from build123d import *

# Parameters (mm, degrees)
BOSS_EXTRUDE1_DEPTH = 15
FILLET1_R           = 30
FILLET2_R           = 6
SKETCH3_W           = 30.5
SKETCH3_H           = 15.5
CUT_EXTRUDE2_DEPTH  = 820.456527218
SKETCH6_W           = 15
SKETCH6_H           = 30
BOSS_EXTRUDE2_DEPTH = 10
SKETCH7_W           = 15
SKETCH7_H           = 15
CUT_EXTRUDE5_DEPTH  = 820.456527218
FILLET4_R           = 6.5
SKETCH9_W           = 75
SKETCH9_H           = 115
BOSS_EXTRUDE3_DEPTH = 15
SKETCH8_W           = 21
SKETCH8_H           = 11
CUT_EXTRUDE6_DEPTH  = 890.119789455
CUT_EXTRUDE7_DEPTH  = 15
SKETCH11_W          = 25
SKETCH11_H          = 50
CUT_EXTRUDE8_DEPTH  = 15
SKETCH5_R           = 2.5
CUT_EXTRUDE4_DEPTH  = 890.119789455
FILLET5_R           = 20
FILLET6_R           = 10
CHAMFER1_SIZE       = 1
SKETCH12_W          = 16
SKETCH12_H          = 11
CUT_EXTRUDE9_DEPTH  = 890.119789455
SKETCH14_W          = 223.5
SKETCH14_H          = 10
CUT_EXTRUDE11_DEPTH = 15
FILLET8_R           = 5
SKETCH15_R          = 2
CUT_EXTRUDE12_DEPTH = 890.119789455
SKETCH16_R          = 2
CUT_EXTRUDE13_DEPTH = 890.119789455
SKETCH17_R          = 2
CUT_EXTRUDE14_DEPTH = 890.119789455
BOSS_EXTRUDE4_DEPTH = 15
FILLET9_R           = 10
FILLET10_R          = 3
SKETCH19_R          = 4.25
CUT_EXTRUDE15_DEPTH = 932.739770537


with BuildPart() as part:
    # Sketch1 → Boss-Extrude1 (new body)
    with BuildSketch(Plane(origin=(0, 0, 0), x_dir=(0, 0, -1), z_dir=(1, 0, 0))):
        Polygon((-678, 0), (0, 0), (0, 460), (75, 460), (75, -69), (-678, -69), align=None)
    extrude(amount=BOSS_EXTRUDE1_DEPTH)

    # Fillet1
    fillet1_edges = [part.edges().sort_by_distance(p)[0] for p in [
        (7.5, -69, -75),
    ]]
    fillet(fillet1_edges, radius=FILLET1_R)

    # Fillet2
    fillet2_edges = [part.edges().sort_by_distance(p)[0] for p in [
        (7.5, 0, 0),
    ]]
    fillet(fillet2_edges, radius=FILLET2_R)

    # Sketch3 → Cut-Extrude2 (cut, through all)
    with BuildSketch(Plane.ZY):
        with Locations((-15.25, 213.5)):
            Rectangle(SKETCH3_W, SKETCH3_H)
    extrude(amount=-CUT_EXTRUDE2_DEPTH, mode=Mode.SUBTRACT)

    # Sketch6 → Boss-Extrude2 (add)
    with BuildSketch(Plane.XY):
        with Locations((7.5, 445)):
            Rectangle(SKETCH6_W, SKETCH6_H)
        with Locations((7.5, 145)):
            Rectangle(SKETCH6_W, SKETCH6_H)
    extrude(amount=BOSS_EXTRUDE2_DEPTH)

    # Sketch7 → Cut-Extrude5 (cut, through all)
    with BuildSketch(Plane.ZY):
        with Locations((-7.5, 198.25)):
            Rectangle(SKETCH7_W, SKETCH7_H)
    extrude(amount=-CUT_EXTRUDE5_DEPTH, mode=Mode.SUBTRACT)

    # Fillet4
    fillet4_edges = [part.edges().sort_by_distance(p)[0] for p in [
        (7.5, 190.75, -15),
    ]]
    fillet(fillet4_edges, radius=FILLET4_R)

    # Sketch9 → Boss-Extrude3 (add)
    with BuildSketch(Plane(origin=(15, 0, 0), x_dir=(0, 0, -1), z_dir=(1, 0, 0))):
        with Locations((37.5, 517.5)):
            Rectangle(SKETCH9_W, SKETCH9_H)
    extrude(amount=-BOSS_EXTRUDE3_DEPTH)

    # Sketch8 → Cut-Extrude6 (cut, through all)
    with BuildSketch(Plane(origin=(15, 0, 0), x_dir=(0, 0, -1), z_dir=(1, 0, 0))):
        with Locations((60, 455)):
            Rectangle(SKETCH8_W, SKETCH8_H)
    extrude(amount=-CUT_EXTRUDE6_DEPTH, mode=Mode.SUBTRACT)

    # Sketch10 → Cut-Extrude7 (cut)
    with BuildSketch(Plane(origin=(15, 0, 0), x_dir=(0, 0, -1), z_dir=(1, 0, 0))):
        Polygon((45, 575), (75, 475), (75, 575), align=None)
    extrude(amount=-CUT_EXTRUDE7_DEPTH, mode=Mode.SUBTRACT)

    # Sketch11 → Cut-Extrude8 (cut)
    with BuildSketch(Plane(origin=(15, 0, 0), x_dir=(0, 0, -1), z_dir=(1, 0, 0))):
        with Locations((27.5, 520)):
            Rectangle(SKETCH11_W, SKETCH11_H)
    extrude(amount=-CUT_EXTRUDE8_DEPTH, mode=Mode.SUBTRACT)

    # Sketch5 → Cut-Extrude4 (cut, through all)
    with BuildSketch(Plane.ZY):
        with Locations((-60, 431)):
            Circle(SKETCH5_R)
    extrude(amount=-CUT_EXTRUDE4_DEPTH, mode=Mode.SUBTRACT)

    # Fillet5
    fillet5_edges = [part.edges().sort_by_distance(p)[0] for p in [
        (7.5, 575, -45),
        (7.5, 475, -75),
    ]]
    fillet(fillet5_edges, radius=FILLET5_R)

    # Fillet6
    fillet6_edges = [part.edges().sort_by_distance(p)[0] for p in [
        (7.5, 495, -15),
        (7.5, 545, -15),
        (7.5, 545, -40),
        (7.5, 495, -40),
    ]]
    fillet(fillet6_edges, radius=FILLET6_R)

    # Chamfer1
    chamfer1_edges = [part.edges().sort_by_distance(p)[0] for p in [
        (7.5, 430, 10),
        (7.5, 460, 10),
        (7.5, 130, 10),
        (7.5, 160, 10),
    ]]
    chamfer(chamfer1_edges, length=CHAMFER1_SIZE)

    # Sketch12 → Cut-Extrude9 (cut, through all)
    with BuildSketch(Plane(origin=(15, 0, 0), x_dir=(0, 0, -1), z_dir=(1, 0, 0))):
        with Locations((27.5, -58.5)):
            Rectangle(SKETCH12_W, SKETCH12_H)
    extrude(amount=-CUT_EXTRUDE9_DEPTH, mode=Mode.SUBTRACT)

    # Sketch14 → Cut-Extrude11 (cut)
    with BuildSketch(Plane(origin=(15, 0, 0), x_dir=(0, 0, -1), z_dir=(1, 0, 0))):
        with Locations((-491.25, -5)):
            Rectangle(SKETCH14_W, SKETCH14_H)
        with Locations((-192.75, -5)):
            Rectangle(SKETCH14_W, SKETCH14_H)
    extrude(amount=-CUT_EXTRUDE11_DEPTH, mode=Mode.SUBTRACT)

    # Fillet8
    fillet8_edges = [part.edges().sort_by_distance(p)[0] for p in [
        (7.5, -10, 603),
        (7.5, -10, 379.5),
        (7.5, -10, 81),
        (7.5, -10, 304.5),
    ]]
    fillet(fillet8_edges, radius=FILLET8_R)

    # Sketch15 → Cut-Extrude12 (cut, through all)
    with BuildSketch(Plane(origin=(15, 0, 0), x_dir=(0, 0, -1), z_dir=(1, 0, 0))):
        with Locations((-0.707106781, 129.292893219)):
            Circle(SKETCH15_R)
        with Locations((-0.707106781, 160.707106781)):
            Circle(SKETCH15_R)
        with Locations((-0.707106781, 429.292893219)):
            Circle(SKETCH15_R)
        with Locations((-0.707106781, 460.707106781)):
            Circle(SKETCH15_R)
    extrude(amount=-CUT_EXTRUDE12_DEPTH, mode=Mode.SUBTRACT)

    # Sketch16 → Cut-Extrude13 (cut, through all)
    with BuildSketch(Plane(origin=(15, 0, 0), x_dir=(0, 0, -1), z_dir=(1, 0, 0))):
        with Locations((50.207106781, 450.207106781)):
            Circle(SKETCH16_R)
        with Locations((50.207106781, 459.792893219)):
            Circle(SKETCH16_R)
        with Locations((69.792893219, 459.792893219)):
            Circle(SKETCH16_R)
        with Locations((69.792893219, 450.207106781)):
            Circle(SKETCH16_R)
    extrude(amount=-CUT_EXTRUDE13_DEPTH, mode=Mode.SUBTRACT)

    # Sketch17 → Cut-Extrude14 (cut, through all)
    with BuildSketch(Plane(origin=(15, 0, 0), x_dir=(0, 0, -1), z_dir=(1, 0, 0))):
        with Locations((29.792893219, 206.457106781)):
            Circle(SKETCH17_R)
        with Locations((29.792893219, 220.542893219)):
            Circle(SKETCH17_R)
    extrude(amount=-CUT_EXTRUDE14_DEPTH, mode=Mode.SUBTRACT)

    # Sketch18 → Boss-Extrude4 (add)
    with BuildSketch(Plane(origin=(15, 0, 0), x_dir=(0, 0, -1), z_dir=(1, 0, 0))):
        with BuildLine():
            Line((-678, -69), (-733, -69))
            Line((-733, -69), (-733, -7))
            Line((-733, -7), (-725.5, -7))
            Line((-725.5, -7), (-720.55324034, -25.378780397))
            ThreePointArc((-720.55324034, -25.378780397), (-708, -35), (-695.44675966, -25.378780397))
            Line((-695.44675966, -25.378780397), (-690.5, -7))
            Line((-690.5, -7), (-678, -7))
            Line((-678, -7), (-678, -69))
        make_face()
    extrude(amount=-BOSS_EXTRUDE4_DEPTH)

    # Fillet9
    fillet9_edges = [part.edges().sort_by_distance(p)[0] for p in [
        (7.5, -69, 733),
    ]]
    fillet(fillet9_edges, radius=FILLET9_R)

    # Fillet10
    fillet10_edges = [part.edges().sort_by_distance(p)[0] for p in [
        (7.5, -7, 733),
        (7.5, -7, 725.5),
        (7.5, -7, 690.5),
    ]]
    fillet(fillet10_edges, radius=FILLET10_R)

    # Sketch19 → Cut-Extrude15 (cut, through all)
    with BuildSketch(Plane(origin=(15, 0, 0), x_dir=(0, 0, -1), z_dir=(1, 0, 0))):
        with Locations((-513, -34)):
            Circle(SKETCH19_R)
        with Locations((-363, -34)):
            Circle(SKETCH19_R)
    extrude(amount=-CUT_EXTRUDE15_DEPTH, mode=Mode.SUBTRACT)


solid = part.part
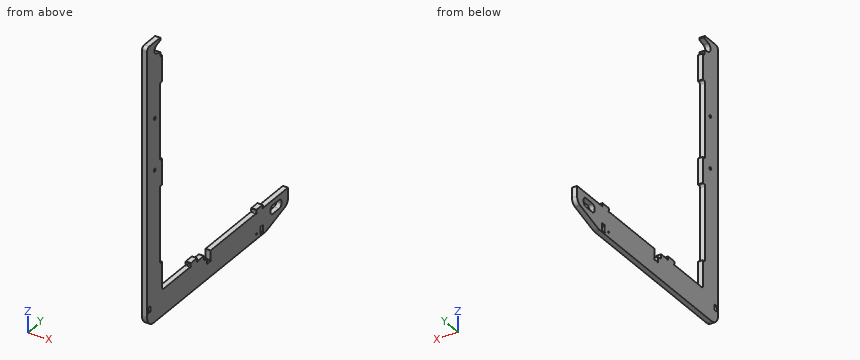
Verification items for the finished model (mm, model axes). Coordinates: 2 decimals unless noted, no trailing zeros. Loops run counter-clockwise (first coordinate to the right, second up) from the corner with the lowest first, then second, coordinate; pieces in that order, holes last. Notation, with made-up numbers: (-16, 47) -> (30, 47) arc R27 ccw to (30, 65) -> close; hole circle Ø2 at (51, 32). An arc over 180 degrees is marked (long way). Answer as a JSON object with one key per item and string values. Group by question number.
Item 1: Depth check by flat-ended pin: pin 1 (2 mm diameter, centred on x = 4, z = 356, fed in from +Y); pin 2 (5 mm diameter, centred on x = 8.5, z = 7, fed in from +Y); pin 3 (4.5 mm diameter, centred on x = 7.5, y = 182.5, fed in from +Z). Enter the tip coordinate at first touch or a pass-through.
Item 2: Sectioned sample at B-B on y = 355. Record the boundary of the cut face in (x, z).
Item 3: Scan lines: probe 1 along Z at (x, y) = (7.5, -3); probe 2 along Z at (x, y) = (3.75, 431); probe 3 along Y at (x, z) = (8.5, 414). Record each from-to range of solid material in increasing order.
Item 4: Sectioned sample at A-A on z = 665. Record the boundary of the cut face in (x, y).
Evaluation:
{
 "1": {"pin 1": "stops at y = 0", "pin 2": "stops at y = 460", "pin 3": "stops at z = 0"},
 "2": {"outline": "(0, -75) -> (15, -75) -> (15, 0) -> (0, 0) -> close"},
 "3": {"probe 1": "z = -75 to 81, 304.5 to 379.5, 603 to 678", "probe 2": "z = -75 to -62.5, -57.5 to -0.33, 1.75 to 10", "probe 3": "y = -69 to -10"},
 "4": {"outline": "(0, -69) -> (15, -69) -> (15, 0) -> (0, 0) -> close"}
}
